Check sheet for the modelled part. Datum: model origin and axes. Units: mm. Face numbers are marked on the shaded views. A direction names the side the tool comes from. Round coordinates to 2 decimals unless told otherwise and drop trailing zeros. Write each loop counter-clockwise with the first axis right and the second up, starting at its lowest first coordinate (ties: lowest second). Pieces come first, ordered by that corner, then holes. Notation, with made-up numbers: (58, 53.25) -> (85, 53.25) arc R23 ccw to (85, 63.25) -> close; hole circle Ø4 at (59.25, -4). An arc over 180 degrees is marked (long way). One line per item, written item: value.
from build123d import *

# Parameters (mm, degrees)
CYLINDER913_R             = 1.5
CYLINDER913_DEPTH         = 5
CYLINDER914_R             = 1.5
CYLINDER914_DEPTH         = 5
CYLINDER915_R             = 1.5
CYLINDER915_DEPTH         = 5
CYLINDER916_R             = 1.5
CYLINDER916_DEPTH         = 5
FUSION064_PLACEMENT_ANGLE = 90
CYLINDER909_R             = 11
CYLINDER909_DEPTH         = 1.5
CYLINDER910_R             = 11
CYLINDER910_DEPTH         = 1.5
CYLINDER908_R             = 9
CYLINDER908_DEPTH         = 2


with BuildPart() as cylinder913:
    # Cylinder913 → Cylinder913 (new body)
    with BuildSketch(Plane(origin=(7, 0, 0), x_dir=(1, 0, 0), z_dir=(0, 0, 1))):
        Circle(CYLINDER913_R)
    extrude(amount=CYLINDER913_DEPTH)


with BuildPart() as fusion063:
    # Cylinder914 → Cylinder914 (new body)
    with BuildSketch(Plane(origin=(-7, 0, 0), x_dir=(1, 0, 0), z_dir=(0, 0, 1))):
        Circle(CYLINDER914_R)
    extrude(amount=CYLINDER914_DEPTH)

    # Fusion063: union Cylinder913
    add(cylinder913.part)


with BuildPart() as cylinder915:
    # Cylinder915 → Cylinder915 (new body)
    with BuildSketch(Plane(origin=(7, 0, 0), x_dir=(1, 0, 0), z_dir=(0, 0, 1))):
        Circle(CYLINDER915_R)
    extrude(amount=CYLINDER915_DEPTH)


with BuildPart() as fusion065:
    # Cylinder916 → Cylinder916 (new body)
    with BuildSketch(Plane(origin=(-7, 0, 0), x_dir=(1, 0, 0), z_dir=(0, 0, 1))):
        Circle(CYLINDER916_R)
    extrude(amount=CYLINDER916_DEPTH)

    # Fusion064: union Cylinder915
    add(cylinder915.part)


with BuildPart() as fusion065_1:
    # Fusion064 placement: moved
    add(fusion065.part.rotate(Axis((0, 0, 0), (0, 0, 1)), FUSION064_PLACEMENT_ANGLE))

    # Fusion065: union Fusion063
    add(fusion063.part)


with BuildPart() as fusion065_2:
    # Fusion065 placement: moved
    add(fusion065_1.part.moved(Location((0, 0, 8))))


with BuildPart() as cylinder909:
    # Cylinder909 → Cylinder909 (new body)
    with BuildSketch(Plane.XY.offset(15.5)):
        Circle(CYLINDER909_R)
    extrude(amount=CYLINDER909_DEPTH)


with BuildPart() as cylinder910:
    # Cylinder910 → Cylinder910 (new body)
    with BuildSketch(Plane.XY.offset(12)):
        Circle(CYLINDER910_R)
    extrude(amount=CYLINDER910_DEPTH)


with BuildPart() as selector_gear:
    # Cylinder908 → Cylinder908 (new body)
    with BuildSketch(Plane.XY.offset(13.5)):
        Circle(CYLINDER908_R)
    extrude(amount=CYLINDER908_DEPTH)

    # Fusion072: union Cylinder909, Cylinder910
    add(cylinder909.part)
    add(cylinder910.part)


with BuildPart() as selector_gear_1:
    # Fusion072 placement: moved
    add(selector_gear.part.moved(Location((0, 0, 1))))

    # Fusion073: union Fusion065
    add(fusion065_2.part)


with BuildPart() as selector_gear_2:
    # Fusion073 placement: moved
    add(selector_gear_1.part.moved(Location((0, 0, -1.5))))


solid = selector_gear_2.part
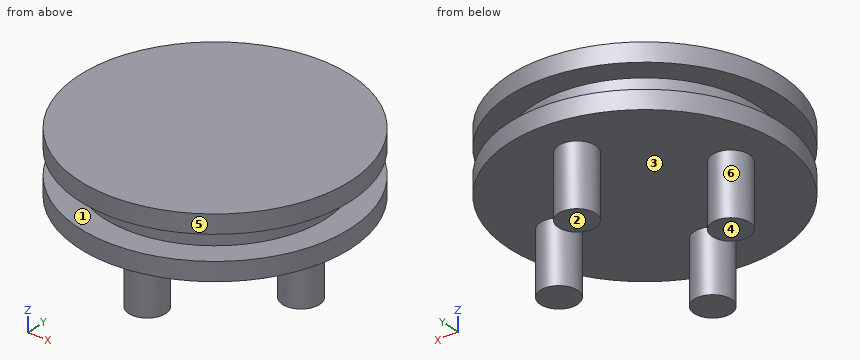
Item 1: Sectioned sample at A-A on z = 10.5. Enter the section's corners in (x, y).
Answer:
outline: circle Ø3 at (-7, 0); circle Ø3 at (0, -7); circle Ø3 at (0, 7); circle Ø3 at (7, 0)
Item 2: Depth check by flat-ended pin: P1, Ø5, axis at x = 4, z = 13.5, coming from the +Y side; P2, Ø3, axis at x = -6.5, z = 8, coming from the +Y side. Enter the tip coordinate at first touch or a pass-through.
Answer:
P1: stops at y = 10.89
P2: stops at y = 1.5
Item 3: Mould release check, pull along X, two halves, no side actions. Record for the marked faces 4, 5 and 6: pulls with the +X half, pulls with the -X half, needs draft (parallel to the pull), parting line crosses it, or undercut.
Answer:
face 4: needs draft
face 5: parting line crosses it
face 6: undercut
Item 4: Sectioned sample at B-B on x = 0. Enter the section's corners in (y, z), and give its area (3 significant figures).
Answer:
outline: (-11, 11.5) -> (-8.5, 11.5) -> (-8.5, 6.5) -> (-5.5, 6.5) -> (-5.5, 11.5) -> (5.5, 11.5) -> (5.5, 6.5) -> (8.5, 6.5) -> (8.5, 11.5) -> (11, 11.5) -> (11, 13) -> (9, 13) -> (9, 15) -> (11, 15) -> (11, 16.5) -> (-11, 16.5) -> (-11, 15) -> (-9, 15) -> (-9, 13) -> (-11, 13) -> close
area: 132 mm^2
Item 5: Tool access check on the marked faces 1, 2 and 3. Record the directions out of +Z, -Z, +X, -X, +Y, -Y that give a thin tool (end or side, any length) a straight path to the whole face; none if there is none.
Answer:
face 1: none
face 2: -Z, +X, -X, +Y, -Y
face 3: -Z
Item 6: Sectioned sample at D-D on y = 2. Enter the section's corners in (x, z).
Answer:
outline: (-10.82, 11.5) -> (10.82, 11.5) -> (10.82, 13) -> (8.77, 13) -> (8.77, 15) -> (10.82, 15) -> (10.82, 16.5) -> (-10.82, 16.5) -> (-10.82, 15) -> (-8.77, 15) -> (-8.77, 13) -> (-10.82, 13) -> close
Item 7: Thickness scan on line 1 (Z direction, x = -3.75, y = -9); line 2 (Z direction, x = 3, y = -6.25); line 3 (Y direction, x = 1, z = 10.25). Record the ranges inside material, lowest first.
Answer:
line 1: z = 11.5 to 13, 15 to 16.5
line 2: z = 11.5 to 16.5
line 3: y = -8.12 to -5.88, 5.88 to 8.12
Item 8: Sectioned sample at C-C on y = 5. Enter the section's corners in (x, z).
Answer:
outline: (-9.8, 11.5) -> (9.8, 11.5) -> (9.8, 13) -> (7.48, 13) -> (7.48, 15) -> (9.8, 15) -> (9.8, 16.5) -> (-9.8, 16.5) -> (-9.8, 15) -> (-7.48, 15) -> (-7.48, 13) -> (-9.8, 13) -> close
